from build123d import *

# Parameters (mm, degrees)
SKETCH_1_W          = 42
SKETCH_1_H          = 25
EXTRUDE_1_DEPTH     = 20
SKETCH_2_W          = 15.2
SKETCH_2_H          = 15.2
CUT_EXTRUDE_1_DEPTH = 53.810983706
EXTRUDE_2_DEPTH     = 25
SKETCH_5_R          = 1.7
CUT_EXTRUDE_2_DEPTH = 57.833088954
FILLET_1_R          = 3
FILLET_3_R          = 1


with BuildPart() as part:
    # 草图1 → 凸台-拉伸1 (new body)
    with BuildSketch(Plane(origin=(0, 0, 0), x_dir=(1, 0, 0), z_dir=(0, 1, 0))):
        with Locations((21, 12.5)):
            Rectangle(SKETCH_1_W, SKETCH_1_H)
    extrude(amount=EXTRUDE_1_DEPTH)

    # 草图2 → 切除-拉伸1 (cut, through all)
    with BuildSketch(Plane.ZY):
        with Locations((-12.5, 7.6)):
            Rectangle(SKETCH_2_W, SKETCH_2_H)
    extrude(amount=-CUT_EXTRUDE_1_DEPTH, mode=Mode.SUBTRACT)

    # 草图4 → 凸台-拉伸2 (add)
    with BuildSketch(Plane.XY):
        Polygon((10.8, 26), (10.8, 20), (0, 20), align=None)
        Polygon((31.2, 20), (31.2, 29), (42, 20), align=None)
    extrude(amount=-EXTRUDE_2_DEPTH)

    # 草图5 → 切除-拉伸2 (cut, through all)
    with BuildSketch(Plane.XY):
        with Locations((6, 7.5)):
            Circle(SKETCH_5_R)
        with Locations((21, 7.5)):
            Circle(SKETCH_5_R)
        with Locations((36, 7.5)):
            Circle(SKETCH_5_R)
    extrude(amount=-CUT_EXTRUDE_2_DEPTH, mode=Mode.SUBTRACT)

    # 圆角1
    fillet_1_edges = [part.edges().sort_by_distance(p)[0] for p in [
        (42, 20, -12.5),
        (0, 0, -2.45),
        (42, 0, -22.55),
        (0, 20, -12.5),
        (42, 0, -2.45),
        (0, 0, -22.55),
    ]]
    fillet(fillet_1_edges, radius=FILLET_1_R)

    # 圆角3
    fillet_3_edges = [part.edges().sort_by_distance(p)[0] for p in [
        (10.8, 26, -12.5),
        (31.2, 29, -12.5),
    ]]
    fillet(fillet_3_edges, radius=FILLET_3_R)


solid = part.part
For this review, take the finished solid that the model builds, in its own axes (mm). A direction names the side the tool comes from. Round coordinates to 2 decimals unless told otherwise and drop trailing zeros. Loops run counter-clockwise (first coordinate to the right, second up) from the corner with the lowest first, then second, coordinate; pieces in that order, holes last. Notation, with made-up numbers: (73, -8.75) - (103, -8.75) arc R33 ccw to (103, 19.25) - close; hole circle Ø8 at (9.5, 59.5). An arc over 180 degrees is marked (long way). One line per item, written item: value. Start each with the question number.
Item 1: For faces 5 (the flat face through (10.8, 22, -12)), 6 (the flat face through (21, 11, 0)), 7 (the flat face through (21, 11, -4.9)), list the 3-axis set-ups (+Z, -Z, +X, -X, +Y, -Y) from which the entire face can be reached by the end or side of a thin tool; tool diameter is ignored.
Item 2: For L1, parallel to Z at x = 25, y = 2.25; L2, parallel to Y at x = 30, z = -9.5; L3, parallel to Y at x = 21, z = -3.2, list the stretches that pass through material, from the lowest coordinate up.
Item 3: Take a section at B-B (y = 7.5). State how many separate pieces and enclosed holes the cut face has, plus the area to 3 significant figures.
Item 4: The part is to be moulded in two halves that separate along X. For faces 1 (the flat face through (21, 0, -2)), 2 (the cylindrical face through (34.65, 6.47, -2.42)), 3 (the flat face through (0, 16, -12)), 4 (the cylindrical face through (5.63, 5.84, -22.52)), say which applies: +X half, -X half, draft (parallel to the pull), parting line (faces both ways), or undercut.
Item 5: Take a section at D-D (z = -9.25). Give the boundary of the cut face in (x, y).
Item 6: Clearance check with flat-ended pins moving along their axes: pin 1 Ø12 at (x, z) = (18, -12.5) entering from -Y; pin 2 Ø3 at (x, z) = (18.5, -3) entering from +Y; pin 3 Ø4 at (x, z) = (34.5, -6.5) entering from +Y. State where each tip first meets the part, or that it passes through.
Item 7: Take a section at C-C (x = 24). Give the boundary of the cut face in (y, z).
Item 8: Take a section at A-A (x = 36). Give the boundary of the cut face in (y, z).
Answer below:
1. face 5: +Z, -Z, +Y
1. face 6: +Z, +X, -X, +Y, -Y
1. face 7: +X, -X, -Y
2. L1: z = -25 to -20.1, -4.9 to 0
2. L2: y = 15.2 to 20
2. L3: y = 0 to 5.8, 9.2 to 20
3. separate pieces: 8
3. enclosed holes: 0
3. area: 312 mm2
4. face 1: draft
4. face 2: undercut
4. face 3: -X half
4. face 4: undercut
5. outline: (0, 15.2) - (42, 15.2) - (42, 18.59) arc R3 ccw to (40.92, 20.9) - (32.84, 27.63) arc R1 ccw to (31.2, 26.86) - (31.2, 20) - (10.8, 20) - (10.8, 24.3) arc R1 ccw to (9.31, 25.17) - (1.54, 20.86) arc R3 ccw to (0, 18.23) - close
6. pin 1: stops at y = 15.2
6. pin 2: stops at y = 20
6. pin 3: stops at y = 27.82
7. outline: (0, -25) - (20, -25) - (20, 0) - (0, 0) - (0, -4.9) - (15.2, -4.9) - (15.2, -20.1) - (0, -20.1) - close
8. outline: (0, -25) - (5.8, -25) - (5.8, -20.1) - (0, -20.1) - close; (0, -4.9) - (5.8, -4.9) - (5.8, 0) - (0, 0) - close; (9.2, -25) - (25, -25) - (25, 0) - (9.2, 0) - (9.2, -4.9) - (15.2, -4.9) - (15.2, -20.1) - (9.2, -20.1) - close
